from build123d import *

# Parameters (mm, degrees)
F0_W     = 177.8
F0_H     = 76.2
F0_W_2   = 3.0734
F0_H_2   = 25.4
F1_DEPTH = 3.0734


with BuildPart() as f1:
    # F0 (on Top) → F1 (new body)
    with BuildSketch(Plane.XY):
        with Locations((18.3134, -0.306201)):
            Rectangle(F0_W, F0_H)
        with Locations((19.8501, -0.306201)):
            Rectangle(F0_W_2, F0_H_2, mode=Mode.SUBTRACT)
        with Locations((-56.3499, -0.306201)):
            Rectangle(F0_W_2, F0_H_2, mode=Mode.SUBTRACT)
        with Locations((-43.6499, -0.306201)):
            Rectangle(F0_W_2, F0_H_2, mode=Mode.SUBTRACT)
        with Locations((96.0501, -0.306201)):
            Rectangle(F0_W_2, F0_H_2, mode=Mode.SUBTRACT)
    extrude(amount=F1_DEPTH)


solid = f1.part
Part model, mm, in its own coordinate system. A direction names the side the tool comes from. Give positions to 0.01 mm unless a question says otherwise; leave off trailing zeros. Write each loop counter-clockwise with the first axis right and the second up, starting at its lowest first coordinate (ties: lowest second). Pieces come first, ordered by that corner, then holes.
1) Probe L1, parallel to X at y = 11, z = 1.65; L2, parallel to Y at x = 18.5, z = 1.5. List the from-to ranges inside material, lowest first.
Resolved:
L1: x = -70.59 to -57.89, -54.81 to -45.19, -42.11 to 18.31, 21.39 to 94.51, 97.59 to 107.21
L2: y = -38.41 to -13.01, 12.39 to 37.79
2) Cut at A-A on y = -3.5. Write the cut outline in (x, z), then the cut area to 3 significant figures.
Resolved:
outline: (-70.59, 0) - (-57.89, 0) - (-57.89, 3.07) - (-70.59, 3.07) - close; (-54.81, 0) - (-45.19, 0) - (-45.19, 3.07) - (-54.81, 3.07) - close; (-42.11, 0) - (18.31, 0) - (18.31, 3.07) - (-42.11, 3.07) - close; (21.39, 0) - (94.51, 0) - (94.51, 3.07) - (21.39, 3.07) - close; (97.59, 0) - (107.21, 0) - (107.21, 3.07) - (97.59, 3.07) - close
area: 509 mm2
3) Cut at B-B on z = 1.85. Write the cut outline in (x, y), then the cut area to 3 significant figures.
Resolved:
outline: (-70.59, -38.41) - (107.21, -38.41) - (107.21, 37.79) - (-70.59, 37.79) - close; hole (-57.89, -13.01) - (-54.81, -13.01) - (-54.81, 12.39) - (-57.89, 12.39) - close; hole (-45.19, -13.01) - (-42.11, -13.01) - (-42.11, 12.39) - (-45.19, 12.39) - close; hole (18.31, -13.01) - (21.39, -13.01) - (21.39, 12.39) - (18.31, 12.39) - close; hole (94.51, -13.01) - (97.59, -13.01) - (97.59, 12.39) - (94.51, 12.39) - close
area: 13,200 mm2
4) Two-plate mould, pull along X, no slides. Class faces 1 (the face through (107.213, -1, 2)), 2 (the face through (17, 37.794, 2)), 3 (the face through (-42.113, 0, 2)): released by +X, released by -X, zero draft, split by the parting line, or undercut.
Resolved:
face 1: released by +X
face 2: zero draft
face 3: undercut
5) Which spindle directions (+Z, -Z, +X, -X, +Y, -Y) get a long thin tool onto all of the face, cutting with end or side? Do faces 4 (the face through (20, 12.394, 2)), 5 (the face through (17, 0, 3.073)). Say none if no direction does.
Resolved:
face 4: +Z, -Z
face 5: +Z, +X, -X, +Y, -Y
